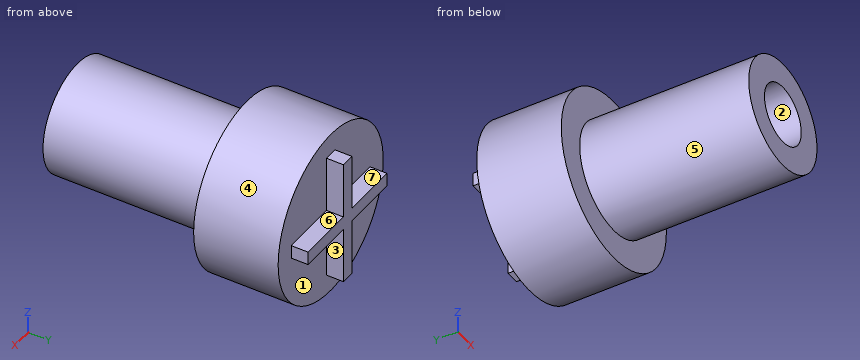
from build123d import *

# Parameters (mm, degrees)
SKETCH1_R           = 3.25
BOSS_EXTRUDE1_DEPTH = 10
SKETCH2_R           = 1.75
CUT_EXTRUDE1_DEPTH  = 2.5
SKETCH6_R           = 5
BOSS_EXTRUDE2_DEPTH = 5
BOSS_EXTRUDE3_DEPTH = 1


with BuildPart() as part:
    # Sketch1 → Boss-Extrude1 (new body)
    with BuildSketch(Plane(origin=(0, 0, 0), x_dir=(1, 0, 0), z_dir=(0, 1, 0))):
        Circle(SKETCH1_R)
    extrude(amount=BOSS_EXTRUDE1_DEPTH)

    # Sketch2 → Cut-Extrude1 (cut)
    with BuildSketch(Plane.XZ):
        Circle(SKETCH2_R)
    extrude(amount=-CUT_EXTRUDE1_DEPTH, mode=Mode.SUBTRACT)

    # Sketch6 → Boss-Extrude2 (add)
    with BuildSketch(Plane(origin=(0, 10, 0), x_dir=(1, 0, 0), z_dir=(0, 1, 0))):
        Circle(SKETCH6_R)
    extrude(amount=BOSS_EXTRUDE2_DEPTH)

    # Sketch8 → Boss-Extrude3 (add)
    with BuildSketch(Plane(origin=(0, 15, 0), x_dir=(1, 0, 0), z_dir=(0, 1, 0))):
        Polygon((0.4, 3.75), (-0.4, 3.75), (-0.4, 0.4), (-3.75, 0.4), (-3.75, -0.4), (-0.4, -0.4), (-0.4, -3.75), (0.4, -3.75), (0.4, -0.4), (3.75, -0.4), (3.75, 0.4), (0.4, 0.4), align=None)
    extrude(amount=BOSS_EXTRUDE3_DEPTH)


solid = part.part
Geometry check sheet. Reference: the model listing, model coordinates, mm. Face numbers are marked on the shaded views. A direction names the side the tool comes from. Give positions to 0.01 mm unless a question says otherwise; leave off trailing zeros. Loops run counter-clockwise (first coordinate to the right, second up) from the corner with the lowest first, then second, coordinate; pieces in that order, holes last. Notation, with made-up numbers: (1.5, -11.5) -> (49.5, -11.5) arc R32 cw to (49.5, 23.5) -> close; hole circle Ø10 at (-12.75, -11). An arc over 180 degrees is marked (long way). Answer in a Markdown table with one row per item. Add a question column.
1) Cross-section at C-C on y = 8.5. Record the boundary of the cut face in (x, z).
2) Set-up check for the marked faces 5, 6 and 7: record each of +Z, -Z, +X, -X, +Y, -Y from which the full face is reachable in a straight line by a thin tool's end or side.
3) Draft check along X on the marked faces 1, 2, 3 and 4. Enter one of: pulls with the +X half, pulls with the -X half, needs draft (parallel to the pull), parting line crosses it, or undercut.
4) Cross-section at A-A on z = 0. Record the boundary of the cut face in (x, y).
5) Material ranges on probe 1 along Z at (x, y) = (0, 1.8); probe 2 along Y at (x, z) = (2, 0.75); probe 3 along Y at (x, z) = (3.75, -1.25), recorded low to high. Write a range as from..to.
6) Cross-section at D-D on z = -3.5. Record the boundary of the cut face in (x, y).
7) Gauge pin test, flat ends, axial feed: P1, Ø0.9, axis at y = 15.5, z = 0, coming from the -X side; P2, Ø0.5, axis at y = 15.5, z = 1.5, coming from the -X side; P3, Ø2, axis at x = -4, y = 12, coming from the -Z side. Record the tip position at first contact, or that the pin passes through.
8) Cross-section at B-B on x = 0. Record the boundary of the cut face in (y, z).
Outcome:
| question | item | result |
|---|---|---|
| 1 | outline | circle Ø6.5 at (0, 0) |
| 2 | face 5 | -Y |
| 2 | face 6 | +Z, +X, +Y |
| 2 | face 7 | +Z, -X, +Y |
| 3 | face 1 | needs draft |
| 3 | face 2 | undercut |
| 3 | face 3 | pulls with the +X half |
| 3 | face 4 | parting line crosses it |
| 4 | outline | (-5, 10) -> (-3.25, 10) -> (-3.25, 0) -> (-1.75, 0) -> (-1.75, 2.5) -> (1.75, 2.5) -> (1.75, 0) -> (3.25, 0) -> (3.25, 10) -> (5, 10) -> (5, 15) -> (3.75, 15) -> (3.75, 16) -> (-3.75, 16) -> (-3.75, 15) -> (-5, 15) -> close |
| 5 | probe 1 | z = -3.25..-1.75, 1.75..3.25 |
| 5 | probe 2 | y = 0..15 |
| 5 | probe 3 | y = 10..15 |
| 6 | outline | (-3.57, 10) -> (3.57, 10) -> (3.57, 15) -> (0.4, 15) -> (0.4, 16) -> (-0.4, 16) -> (-0.4, 15) -> (-3.57, 15) -> close |
| 7 | P1 | stops at x = -3.75 |
| 7 | P2 | stops at x = -0.4 |
| 7 | P3 | stops at z = -4 |
| 8 | outline | (0, -3.25) -> (10, -3.25) -> (10, -5) -> (15, -5) -> (15, -3.75) -> (16, -3.75) -> (16, 3.75) -> (15, 3.75) -> (15, 5) -> (10, 5) -> (10, 3.25) -> (0, 3.25) -> (0, 1.75) -> (2.5, 1.75) -> (2.5, -1.75) -> (0, -1.75) -> close |
